Input: part model. Units: mm. Frame: model coordinates. Give positions to 0.01 mm unless a question says otherwise; leave off trailing zeros. Write each loop counter-clockwise with the first axis right and the second up, starting at its lowest first coordinate (ties: lowest second). Pieces come first, ordered by that corner, then holes. Notation, with made-up numbers: (-17, 84.5) -> (18, 84.5) arc R10 cw to (18, 95.5) -> close; hole circle Ø1 at (-24.5, -32.75). An arc over 180 degrees is marked (long way). Return JSON: item names as keys, results as strings. Group by question number.
Item 1: Mould query, pull axis X, two halves, no side actions, for faces 1 (the face through (-5.771, -16.136, 1.61)), 2 (the face through (-18.941, 9.615, 1.565)), 3 (the face through (-0.17, 19.05, 1.57)), 4 (the face through (-13.68, 0.24, 1.61)). Classes: released by +X, released by -X, zero draft, split by the parting line, or undercut.
Item 2: Line query: line 1 (Y direction, x = 0, z = 1.45); line 2 (Y direction, x = -10, z = 0.5) (3 decimals); line 3 (Y direction, x = -15, z = 0.9). Output: solid intervals per line, ascending. Write a range as [from, to].
Item 3: Pin query (flat end, axial travel): P1, Ø1, axis at y = 7.5, z = 1, coming from the -X side; P2, Ø1, axis at x = -13.5, z = 1, coming from the -Y side; P3, Ø1, axis at y = 2, z = 1.5, coming from the +X side. Return the tip coordinate at first contact, or that it passes through.
Item 4: Section B-B, the plane x = 0. Return loops of the section in (y, z) (1 decimal).
Item 5: Section A-A, the plane y = 0. Return loops of the section in (x, z) (1 decimal).
Autodesk Inventor part; units mm, degrees
ref_plane "YZ Plane" through (0, 0, 0) normal (1, 0, 0) x (0, 1, 0)
ref_plane "XZ Plane" through (0, 0, 0) normal (0, 1, 0) x (-1, 0, 0)
ref_plane "XY Plane" through (0, 0, 0) normal (0, 0, 1) x (1, 0, 0)
sketch "Sketch1" plane through (0, 0, 0) normal (0, 0, 1) x (1, 0, 0)
  line L0 (-11.4198, 15.2476) -> (-26.6751, 3.8221)
  line L1 (-26.6751, -3.8221) -> (-11.4198, -15.2476)
  line L2 (11.4198, 15.2476) -> (26.6751, 3.8221)
  line L3 (26.6751, -3.8221) -> (11.4198, -15.2476)
  line L4 (-31.7782, 0) -> (31.7782, 0) construction
  arc A0 (-26.6751, 3.8221) -> (-26.6751, -3.8221) centre (-23.8125, 0) ccw
  arc A1 (26.6751, -3.8221) -> (26.6751, 3.8221) centre (23.8125, 0) ccw
  arc A2 (-11.4198, -15.2476) -> (11.4198, -15.2476) centre (0, 0) ccw
  arc A3 (11.4198, 15.2476) -> (-11.4198, 15.2476) centre (0, 0) ccw
  dimension "d1" = 4.7752
  dimension "d2" = 47.625
extrude "Extrusion1" add sketch "Sketch1" along normal blind 3.175
sketch "Sketch2" plane through (0, 0, 3.175) normal (0, 0, 1) x (1, 0, 0)
  arc A0 (-26.6751, 3.8221) -> (-26.6751, -3.8221) centre (-23.8125, 0) ccw
  arc A1 (26.6751, -3.8221) -> (26.6751, 3.8221) centre (23.8125, 0) ccw
  circle A2 centre (-23.8125, 0) radius 2.4892
  circle A3 centre (23.8125, 0) radius 2.4892
  circle A4 centre (0, 0) radius 11.1125
  dimension "d5" = 22.225
  dimension "d6" = 4.9784
extrude "Extrusion2" cut sketch "Sketch2" against normal blind 3.175
sketch "Sketch3" plane through (0, 0, 3.175) normal (0, 0, 1) x (1, 0, 0)
  arc A0 (11.4198, 15.2476) -> (-11.4198, 15.2476) centre (0, 0) ccw
  line L0 (0, 19.05) -> (0, -19.6536) construction
  circle A1 centre (0, 15.494) radius 1.8288
  circle A2 centre (0, -15.494) radius 1.8288
  dimension "d9" = 30.988
  dimension "d10" = 15.494
  dimension "d11" = 3.6576
extrude "Extrusion3" cut sketch "Sketch3" against normal blind 3.175
pattern_circular "Circular Pattern1" count 5 over 90 about axis through (0, 0, 3.175) along (0, 0, -1) of "Extrusion3"
properties part number "Pancake Mount Plate" material "Steel, Galvanized"
Answer below:
{
 "1": {"face 1": "undercut", "face 2": "released by -X", "face 3": "split by the parting line", "face 4": "undercut"},
 "2": {"line 1": "y = [-19.05, -17.32], [-13.67, -11.11], [11.11, 13.67], [17.32, 19.05]", "line 2": "y = [-16.214, -12.515], [-9.397, -4.846], [4.846, 16.214]", "line 3": "y = [-12.57, -7.62], [-4.23, -1.76], [1.76, 12.57]"},
 "3": {"P1": "stops at x = -22.43", "P2": "stops at y = -14.06", "P3": "stops at x = 28.35"},
 "4": {"outline": "(-19, 0) -> (-17.3, 0) -> (-17.3, 3.2) -> (-19, 3.2) -> close; (-13.7, 0) -> (-11.1, 0) -> (-11.1, 3.2) -> (-13.7, 3.2) -> close; (11.1, 0) -> (13.7, 0) -> (13.7, 3.2) -> (11.1, 3.2) -> close; (17.3, 0) -> (19, 0) -> (19, 3.2) -> (17.3, 3.2) -> close"},
 "5": {"outline": "(-28.6, 0) -> (-26.3, 0) -> (-26.3, 3.2) -> (-28.6, 3.2) -> close; (-21.3, 0) -> (-17.3, 0) -> (-17.3, 3.2) -> (-21.3, 3.2) -> close; (-13.7, 0) -> (-11.1, 0) -> (-11.1, 3.2) -> (-13.7, 3.2) -> close; (11.1, 0) -> (13.7, 0) -> (13.7, 3.2) -> (11.1, 3.2) -> close; (17.3, 0) -> (21.3, 0) -> (21.3, 3.2) -> (17.3, 3.2) -> close; (26.3, 0) -> (28.6, 0) -> (28.6, 3.2) -> (26.3, 3.2) -> close"}
}
